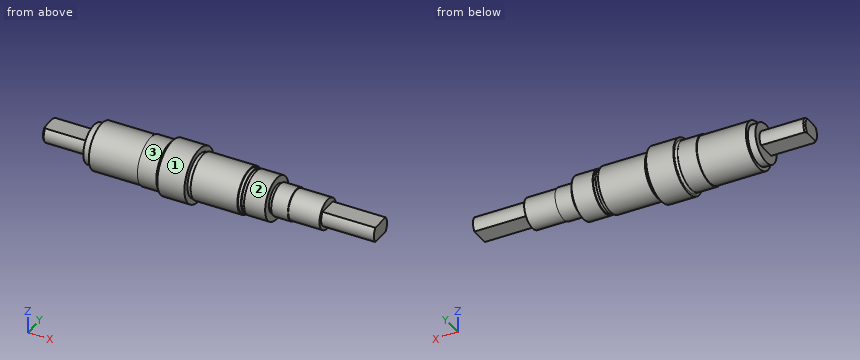
Autodesk Inventor part; units mm, degrees
ref_plane "YZ Plane" through (0, 0, 0) normal (1, 0, 0) x (0, 1, 0)
ref_plane "XZ Plane" through (0, 0, 0) normal (0, 1, 0) x (-1, 0, 0)
ref_plane "XY Plane" through (0, 0, 0) normal (0, 0, 1) x (1, 0, 0)
sketch "Esquisse1" plane through (0, 0, 0) normal (0, 0, 1) x (1, 0, 0)
  line L0 (-110, 0) -> (-110, 7)
  line L1 (-110, 7) -> (-109, 8)
  line L2 (-109, 8) -> (-80, 8)
  line L3 (-80, 8) -> (-80, 13)
  line L4 (-80, 13) -> (-75, 13)
  line L5 (-75, 13) -> (-75, 15.5)
  line L6 (-75, 15.5) -> (-42.5, 15.5)
  line L7 (-110, 0) -> (110, 0)
  line L8 (-42.5, 15.5) -> (-42.5, 16)
  line L9 (-42.5, 16) -> (-30, 16)
  arc A0 (-30, 16) -> (-28.25, 16.5) centre (-29.1964, 16.5) ccw
  line L10 (-28.25, 16.5) -> (-28.25, 18)
  line L11 (-28.25, 18) -> (-10.25, 18)
  line L12 (-10.25, 18) -> (-10.25, 14.25)
  line L13 (-10.25, 14.25) -> (-7.75, 14.25)
  line L14 (-7.75, 14.25) -> (-7.75, 15)
  line L15 (-7.75, 15) -> (23.25, 15)
  line L16 (23.25, 15) -> (23.25, 14.25)
  line L17 (23.25, 14.25) -> (25.25, 14.25)
  line L18 (25.25, 14.25) -> (25.25, 13.5)
  line L19 (25.25, 13.5) -> (27.25, 13.5)
  line L20 (27.25, 13.5) -> (27.25, 14.25)
  line L21 (27.25, 14.25) -> (41.25, 14.25)
  line L22 (41.25, 14.25) -> (41.25, 9.5)
  line L23 (41.25, 9.5) -> (43.25, 9.5)
  line L24 (43.25, 9.5) -> (43.25, 10.5)
  line L25 (43.25, 10.5) -> (54.25, 10.5)
  line L26 (54.25, 10.5) -> (54.25, 10)
  line L27 (54.25, 10) -> (75, 10)
  line L28 (75, 10) -> (75, 8)
  line L29 (75, 8) -> (110, 8)
  line L30 (110, 8) -> (110, 0)
  point P0 (0, 0)
  dimension "d0" = 35
  dimension "d1" = 1
  dimension "d2" = 1
  dimension "d3" = 8
  dimension "d4" = 30
  dimension "d5" = 13
  dimension "d6" = 15.5
  dimension "d7" = 16
  dimension "d8" = 32.5
  dimension "d9" = 12.5
  dimension "d10" = 14.25
  dimension "d11" = 0.5
  dimension "d12" = 18
  dimension "d13" = 18
  dimension "d14" = 14.25
  dimension "d15" = 2.5
  dimension "d16" = 75
  dimension "d17" = 15
  dimension "d18" = 31
  dimension "d19" = 2
  dimension "d20" = 2
  dimension "d21" = 14.25
  dimension "d22" = 13.5
  dimension "d23" = 14.25
  dimension "d24" = 14
  dimension "d25" = 9.5
  dimension "d26" = 2
  dimension "d27" = 75
  dimension "d28" = 10.5
  dimension "d29" = 11
  dimension "d30" = 10
  dimension "d31" = 220
  dimension "d32" = 8
revolve "Révolution1" add sketch "Esquisse1" angle 360 about axis through (-110, 0, 0) along (1, 0, 0)
thread "Filetage1"
sketch "Esquisse2" plane through (-110, 0, 0) normal (-1, 0, 0) x (0, 0, 1)
  circle A0 centre (0, 0) radius 9.5
  line L0 (5, -8.0777) -> (-5, -8.0777)
  line L1 (-5, -8.0777) -> (-5, 8.0777)
  line L2 (-5, 8.0777) -> (5, 8.0777)
  line L3 (5, 8.0777) -> (5, -8.0777)
  line L4 (5, -8.0777) -> (-5, 8.0777) construction
  line L5 (-5, -8.0777) -> (5, 8.0777) construction
  dimension "d34" = 10
extrude "Extrusion1" cut sketch "Esquisse2" against normal up to surface (30 mm away) contours A0 L3 | L2 A0 | A0 L0 | L1 A0
thread "Filetage4"
sketch "Esquisse3" plane through (110, 0, 0) normal (1, 0, 0) x (0, 0, -1)
  line L0 (5, -8.6603) -> (-5, -8.6603)
  line L1 (-5, -8.6603) -> (-5, 8.6603)
  line L2 (-5, 8.6603) -> (5, 8.6603)
  line L3 (5, 8.6603) -> (5, -8.6603)
  line L4 (5, -8.6603) -> (-5, 8.6603) construction
  line L5 (-5, -8.6603) -> (5, 8.6603) construction
  circle A0 centre (0, 0) radius 10
  dimension "d45" = 10
extrude "Extrusion2" cut sketch "Esquisse3" against normal up to surface (35 mm away) contours A0 L0 | L3 A0 | A0 L1 | L2 A0
properties part number "Stator_Axis"
Geometry: final body of the model. Coordinates: model frame, mm. Face numbers are marked on the shaded views. A direction names the side the tool comes from. Coordinates: 2 decimals unless noted, no trailing zeros. Loops run counter-clockwise (first coordinate to the right, second up) from the corner with the lowest first, then second, coordinate; pieces in that order, holes last. Notation, with made-up numbers: (56.5, 78) - (108.5, 78) arc R18 ccw to (108.5, 110) - close; hole circle Ø11 at (50, 82). An arc over 180 degrees is marked (long way). One line per question, with ' | ' between items. Start each with the question number.
(1) Cut plane A-A on x = -55. Output: boundary loops of the cut face in (y, z), and give its area (3 significant figures).
(2) Cut plane B-B on x = 58. Output: boundary loops of the cut face in (y, z), and give its area (3 significant figures).
(3) Reachability of the marked faces 1, 2 and 3 from +Z, -Z, +X, -X, +Y, -Y: full face, straight path, thin tool, end or side. Return the list, or none.
(4) First-contact query: pin 1 (5 mm diameter, centred on x = -24, y = -0.5, fed in from -Z); pin 2 (8 mm diameter, centred on y = -13.5, z = 7, fed in from -X); pin 3 (3.5 mm diameter, centred on x = -91, y = -2, fed in from +Z). Flat tips, straight axial feed; report the tip coordinate or a pass-through.
(5) Ray query, L1, parallel to Z at x = -36, y = 5.5; L2, parallel to X at y = 2.5, z = 8.5; L3, parallel to X at y = 13.5, z = -5.5. Return the intervals inside material, ascending. Write a range as from..to.
Here are the results:
1) outline: circle Ø31 at (0, 0) | area: 755 mm²
2) outline: circle Ø20 at (0, 0) | area: 314 mm²
3) face 1: +X, -X | face 2: +X | face 3: -X
4) pin 1: z = -18 | pin 2: x = -80 | pin 3: z = 5
5) L1: -15.02..15.02 | L2: -80..75 | L3: -75..-10.25, -7.75..23.25
